Here's how the part is built. I have some questions about the finished solid (model axes, mm). A direction names the side the tool comes from. Round coordinates to 2 decimals unless told otherwise and drop trailing zeros. Loops run counter-clockwise (first coordinate to the right, second up) from the corner with the lowest first, then second, coordinate; pieces in that order, holes last. Notation, with made-up numbers: M 52.5,18 L 72.5,18 A28 ccw 72.5,50 Z; hole C -1,38 d7. An arc over 180 degrees is marked long. Answer as CSV lines item,"result".
```python
from build123d import *

# Parameters (mm, degrees)
BOSS_EXTRUDE1_DEPTH     = 20
CUT_EXTRUDE1_DEPTH      = 84.216584885
CUT_EXTRUDE1_DEPTH_BACK = 84.216584885
SKETCH2_W               = 0.5
SKETCH2_H               = 10
CUT_EXTRUDE2_DEPTH      = 135.907375632
CUT_EXTRUDE2_DEPTH_BACK = 135.907375632
SKETCH3_R               = 1.6
CUT_EXTRUDE3_DEPTH      = 84.216584885
CUT_EXTRUDE3_DEPTH_BACK = 84.216584885
SKETCH4_W               = 50
SKETCH4_H               = 2
SKETCH5_R               = 2.5
CUT_EXTRUDE4_DEPTH      = 10


with BuildPart() as part:
    # Sketch1 → Boss-Extrude1 (new body)
    with BuildSketch(Plane(origin=(0, 0, 0), x_dir=(1, 0, 0), z_dir=(0, 1, 0))):
        Polygon((0, 0), (-75, 0), (-75, -20), (-55, -20), (-55, -30), (-45, -30), (-45, -20), (-30, -20), (-30, -30), (-20, -30), (-20, -20), (20, -20), (20, -30), (30, -30), (30, -20), (45, -20), (45, -30), (55, -30), (55, -20), (75, -20), (75, 0), align=None)
    extrude(amount=BOSS_EXTRUDE1_DEPTH)

    # Sketch2 → Cut-Extrude1 (cut, two sides: drawn at the far end of the back side and taken through both)
    with BuildSketch(Plane(origin=(0, 20, 0), x_dir=(1, 0, 0), z_dir=(0, 1, 0)).offset(-CUT_EXTRUDE1_DEPTH_BACK)):
        with Locations((-50, -25)):
            Rectangle(SKETCH2_W, SKETCH2_H)
        with Locations((-25, -25)):
            Rectangle(SKETCH2_W, SKETCH2_H)
        with Locations((25, -25)):
            Rectangle(SKETCH2_W, SKETCH2_H)
        with Locations((50, -25)):
            Rectangle(SKETCH2_W, SKETCH2_H)
    extrude(amount=CUT_EXTRUDE1_DEPTH + CUT_EXTRUDE1_DEPTH_BACK, mode=Mode.SUBTRACT)

    # Sketch3 → Cut-Extrude2 (cut, two sides: drawn at the far end of the back side and taken through both)
    with BuildSketch(Plane.ZY.offset(55).offset(-CUT_EXTRUDE2_DEPTH_BACK)):
        with Locations((25, 15)):
            Circle(SKETCH3_R)
        with Locations((25, 5)):
            Circle(SKETCH3_R)
    extrude(amount=CUT_EXTRUDE2_DEPTH + CUT_EXTRUDE2_DEPTH_BACK, mode=Mode.SUBTRACT)

    # Sketch4 → Cut-Extrude3 (cut, two sides: drawn at the far end of the back side and taken through both)
    with BuildSketch(Plane(origin=(0, 20, 0), x_dir=(1, 0, 0), z_dir=(0, 1, 0)).offset(-CUT_EXTRUDE3_DEPTH_BACK)):
        with Locations((0, -6)):
            Rectangle(SKETCH4_W, SKETCH4_H)
    extrude(amount=CUT_EXTRUDE3_DEPTH + CUT_EXTRUDE3_DEPTH_BACK, mode=Mode.SUBTRACT)

    # Sketch5 → Cut-Extrude4 (cut)
    with BuildSketch(Plane.XY.offset(20)):
        with Locations((0, 5)):
            Circle(SKETCH5_R)
    extrude(amount=-CUT_EXTRUDE4_DEPTH, mode=Mode.SUBTRACT)


solid = part.part
```
1. Which directions (+Z, -Z, +X, -X, +Y, -Y) give clear straight access to the entire face, cutting with the end or side of a thin tool? Please do faces 4 (the flat face through (0, 10, 20)), 5 (the cylindrical face through (-52.59, 4.03, 23.73)).
Evaluation:
face 4,"+Z, +Y, -Y"
face 5,"+X, -X"
2. We'd pull the mould along Y, two halves only. Please class faces 1 (the flat face through (-38, 10, 20)), 2 (the cylindrical face through (47.41, 4.03, 23.73)), 3 (the flat face through (-1, 20, 11)): pulls with the +Y half, pulls with the -Y half, needs draft (parallel to the pull), parting line crosses it, or undercut.
Evaluation:
face 1,"needs draft"
face 2,"undercut"
face 3,"pulls with the +Y half"
3. For P1, Ø4.5, axis at x = 40.5, y = 14.5, coming from the +Z side; P2, Ø5, axis at y = 15, z = 24.5, coming from the +X side; P3, Ø3, axis at y = 15, z = 25, coming from the +X side; P4, Ø11, axis at y = 11, z = 26, coming from the -X side, each with a flat end and sliding along its axis, tell me the tip position at first contact or that it passes through.
Evaluation:
P1,"stops at z = 20"
P2,"stops at x = 55"
P3,"passes through"
P4,"stops at x = -55"
4. If I drill on line 1 (Y direction, x = 53.35, z = 25); line 2 (Z direction, x = -23.05, y = 5); line 3 (Z direction, x = -52.4, y = 5), over which ranges is the centre line in solid material (lowest first)? Write a range as [from, to].
Evaluation:
line 1,"y = [0, 3.4], [6.6, 13.4], [16.6, 20]"
line 2,"z = [0, 5], [7, 23.4], [26.6, 30]"
line 3,"z = [0, 23.4], [26.6, 30]"
5. I want a section at A-A, the plane z = 21.75. Count the separate pieces of the cut face and the enclosed holes in it, and give its area (3 significant figures).
Evaluation:
separate pieces,"8"
enclosed holes,"0"
area,"760 mm²"
6. I want a section at B-B, the plane x = 53.5. Please give me the cut outline in (y, z), and give its area (3 significant figures).
Evaluation:
outline,"M 0,0 L 20,0 L 20,30 L 0,30 Z; hole C 5,25 d3.2; hole C 15,25 d3.2"
area,"584 mm²"
